from build123d import *

# Parameters (mm, degrees)
F0_W     = 86.4
F0_H     = 48.33
F1_DEPTH = 1.61
F3_D     = 4.1
F4_W     = 58.3
F4_H     = 9
F5_DEPTH = 9
F6_W     = 5.8
F6_H     = 18
F7_DEPTH = 12.9
F8_W     = 10.2
F8_H     = 6
F9_DEPTH = 10.2


with BuildPart() as f1:
    # F0 (on Top) → F1 (new body)
    with BuildSketch(Plane.XY):
        with Locations((-43.2, 24.165)):
            Rectangle(F0_W, F0_H)
    extrude(amount=F1_DEPTH)

    # F3 (through all)
    with Locations(Plane.XY.offset(1.61)):
        with Locations((-81.2, 43.33), (-5.1, 43.33), (-5.1, 5.13), (-81.2, 5.13)):
            Hole(F3_D / 2)

    # F4 (on face) → F5 (join)
    with BuildSketch(Plane.XY.offset(1.61)):
        with Locations((-43.05, 41.83)):
            Rectangle(F4_W, F4_H)
    extrude(amount=F5_DEPTH)

    # F6 (on face) → F7 (join)
    with BuildSketch(Plane.XY.offset(1.61)):
        with Locations((-7.6, 23.43)):
            Rectangle(F6_W, F6_H)
    extrude(amount=F7_DEPTH)

    # F8 (on face) → F9 (join)
    with BuildSketch(Plane.XY.offset(1.61)):
        with Locations((-23.4, 5.6)):
            Rectangle(F8_W, F8_H)
        with Locations((-23.4, 23.05)):
            Rectangle(F8_W, F8_H)
        with Locations((-37.433333, 5.6)):
            Rectangle(F8_W, F8_H)
        with Locations((-37.433333, 23.05)):
            Rectangle(F8_W, F8_H)
        with Locations((-51.466667, 5.6)):
            Rectangle(F8_W, F8_H)
        with Locations((-51.466667, 23.05)):
            Rectangle(F8_W, F8_H)
        with Locations((-65.5, 5.6)):
            Rectangle(F8_W, F8_H)
        with Locations((-65.5, 23.05)):
            Rectangle(F8_W, F8_H)
    extrude(amount=F9_DEPTH)


solid = f1.part
Could you check a few things on this model? Use its own coordinates, in mm. A direction names the side the tool comes from. Give positions to 0.01 mm unless a question says otherwise; leave off trailing zeros. Order: outer loops, then holes, each group sorted by start corner. A loop starts at its lowest first (then second) coordinate and runs counter-clockwise, first axis right, second up. Notation, with made-up numbers: (41, 12) - (58, 12) arc R21 cw to (58, 23) - close; hole circle Ø10 at (77, 16.5). An arc over 180 degrees is marked (long way). Return JSON: item names as keys, results as strings. Group by question number.
Q1. Which directions (+Z, -Z, +X, -X, +Y, -Y) give clear straight access to the entire face, cutting with the end or side of a thin tool? Please do faces 4 (the face through (-28.5, 23, 7)), 5 (the face through (-13.9, 42, 6)), 6 (the face through (-52, 26.05, 7)), 7 (the face through (-38, 8.6, 7)).
Q2. Suppose I cut it at D-D, the plane z = 9.75. State how many separate pieces and enclosed holes the cut face has, and give its area (3 significant figures).
Q3. Please list where these lines run through material, in increasing order: line 1 along X through (y, z) = (8.5, 9.5); line 2 along Y through (x, z) = (-81.2, 0.65); line 3 along Y through (x, z) = (-52.5, 3.5). Write a range as [from, to].
Q4. Suppose I cut it at C-C, the plane y = 21. Please give me the cut outline in (x, z), and give its area (3 significant figures).
Q5. Will these pins go through, and if not, where does the flat tip stop? pin 1 Ø1.5 at (x, z) = (-48, 5.5) entering from -Y; pin 2 Ø5 at (x, y) = (-16.5, 27.5) entering from -Z; pin 3 Ø2.5 at (x, z) = (-39, 4) entering from +Y; pin 4 Ø4 at (y, z) = (26, 8) entering from +X.
Q6. Thinking about a two-plate mould opening in Y: for faces 1 (the face through (-70.6, 6, 7)), 2 (the face through (-23, 2.6, 7)), 3 (the face through (-66, 26.05, 7)), which applies, pulls with the +Y half, pulls with the -Y half, needs draft (parallel to the pull), parting line crosses it, or undercut?
Q7. Suppose I cut it at B-B, the plane y = 5.13. Please give me the cut outline in (x, z), and give its area (3 significant figures).
Q8. Suppose I cut it at A-A, the plane x = -81.2. Please give me the cut outline in (y, z).
Resolved:
{
 "1": {"face 4": "+Z, -Y", "face 5": "+Z, +X, +Y, -Y", "face 6": "+Z, -X", "face 7": "+Z, +X, -X"},
 "2": {"separate pieces": "10", "enclosed holes": "0", "area": "1,120 mm2"},
 "3": {"line 1": "x = [-70.6, -60.4], [-56.57, -46.37], [-42.53, -32.33], [-28.5, -18.3]", "line 2": "y = [0, 3.08], [7.18, 41.28], [45.38, 48.33]", "line 3": "y = [2.6, 8.6], [20.05, 26.05], [37.33, 46.33]"},
 "4": {"outline": "(-86.4, 0) - (0, 0) - (0, 1.61) - (-4.7, 1.61) - (-4.7, 14.51) - (-10.5, 14.51) - (-10.5, 1.61) - (-18.3, 1.61) - (-18.3, 11.81) - (-28.5, 11.81) - (-28.5, 1.61) - (-32.33, 1.61) - (-32.33, 11.81) - (-42.53, 11.81) - (-42.53, 1.61) - (-46.37, 1.61) - (-46.37, 11.81) - (-56.57, 11.81) - (-56.57, 1.61) - (-60.4, 1.61) - (-60.4, 11.81) - (-70.6, 11.81) - (-70.6, 1.61) - (-86.4, 1.61) - close", "area": "630 mm2"},
 "5": {"pin 1": "stops at y = 2.6", "pin 2": "stops at z = 0", "pin 3": "stops at y = 46.33", "pin 4": "stops at x = -4.7"},
 "6": {"face 1": "needs draft", "face 2": "pulls with the -Y half", "face 3": "undercut"},
 "7": {"outline": "(-86.4, 0) - (-83.25, 0) - (-83.25, 1.61) - (-86.4, 1.61) - close; (-79.15, 0) - (-7.15, 0) - (-7.15, 1.61) - (-18.3, 1.61) - (-18.3, 11.81) - (-28.5, 11.81) - (-28.5, 1.61) - (-32.33, 1.61) - (-32.33, 11.81) - (-42.53, 11.81) - (-42.53, 1.61) - (-46.37, 1.61) - (-46.37, 11.81) - (-56.57, 11.81) - (-56.57, 1.61) - (-60.4, 1.61) - (-60.4, 11.81) - (-70.6, 11.81) - (-70.6, 1.61) - (-79.15, 1.61) - close; (-3.05, 0) - (0, 0) - (0, 1.61) - (-3.05, 1.61) - close", "area": "542 mm2"},
 "8": {"outline": "(0, 0) - (3.08, 0) - (3.08, 1.61) - (0, 1.61) - close; (7.18, 0) - (41.28, 0) - (41.28, 1.61) - (7.18, 1.61) - close; (45.38, 0) - (48.33, 0) - (48.33, 1.61) - (45.38, 1.61) - close"}
}
